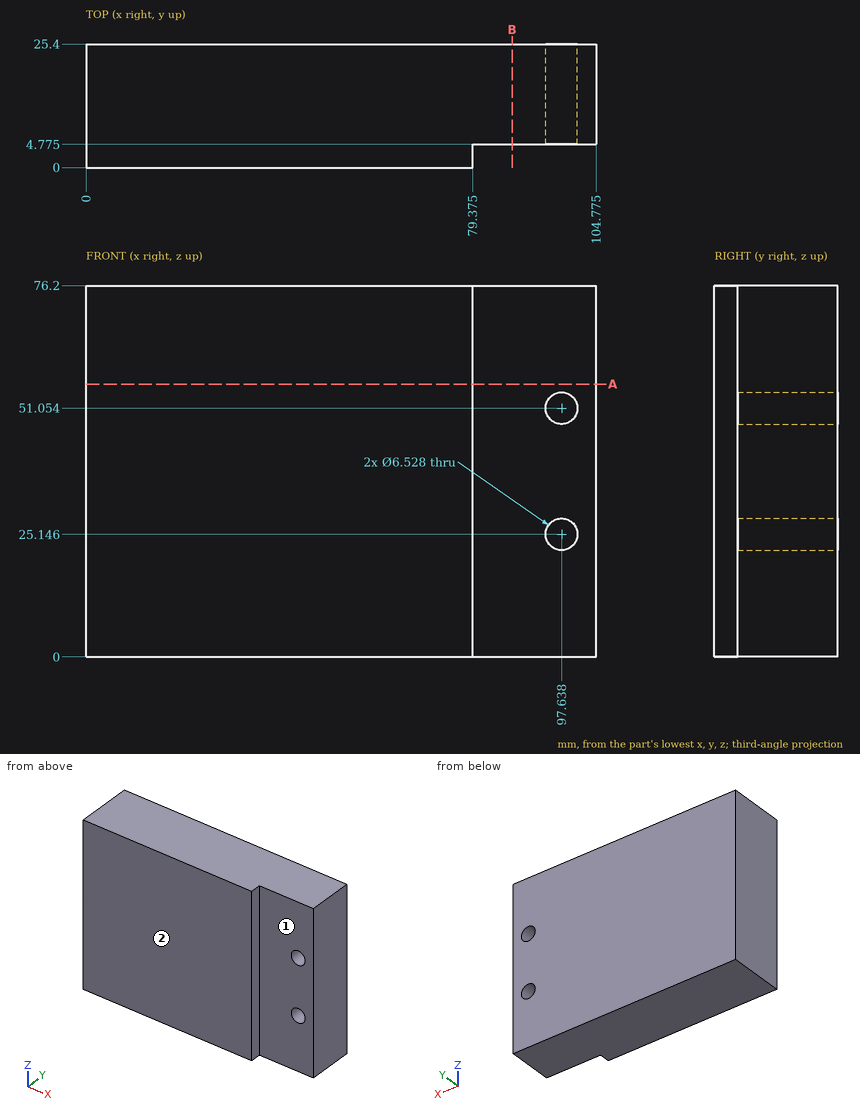
Job drawing, mm, ordinate dimensions from the low corner. One solid piece. A direction names the side the tool comes from. Give positions to 0.01 mm unless a question says otherwise; leave off trailing zeros. Loops run counter-clockwise (first coordinate to the right, second up) from the corner with the lowest first, then second, coordinate; pieces in that order, holes last. Notation, with made-up numbers: M -10.75,-21 L 0.25,-21 A19 cw 0.25,8 Z; hole C 9,-38.75 d7. An arc over 180 degrees is marked long. Return JSON: item names as keys, results as strings.
1) Flat gauge pins, fed straight in: pin 1 Ø8 at (x, y) = (74, 4.5) entering from -Z; pin 2 Ø7.5 at (x, z) = (96, 56) entering from -Y (1 decimal); pin 3 Ø2.5 at (y, z) = (3, 42) entering from +X (3 decimals). Where does each tip first touch, or does it go through?
Calculated:
{"pin 1": "stops at z = 0", "pin 2": "stops at y = 4.8", "pin 3": "stops at x = 79.375"}
2) Saw through at A-A, the plane z = 56. List the corners of the cut face in (x, y) (1 decimal), then the cut area to 3 significant figures.
Calculated:
{"outline": "M 0,0 L 79.4,0 L 79.4,4.8 L 104.8,4.8 L 104.8,25.4 L 0,25.4 Z", "area": "2,540 mm2"}
3) Saw through at B-B, the plane x = 87.5. List the corners of the cut face in (y, z) (1 decimal).
Calculated:
{"outline": "M 4.8,0 L 25.4,0 L 25.4,76.2 L 4.8,76.2 Z"}
4) Drill centre lines: line 1 (X direction, y = 24, z = 51) (1 decimal); line 2 (X direction, y = 4, z = 45) (1 decimal); line 3 (Y direction, x = 87.5, z = 30) (1 decimal). Where is each one in solid material? Low to high.
Calculated:
{"line 1": "x = 0 to 94.4, 100.9 to 104.8", "line 2": "x = 0 to 79.4", "line 3": "y = 4.8 to 25.4"}
5) 3-axis set-ups, long thin cutter, end or side, ignore diameter. For the marked faces 1 and 2: which of +Z, -Z, +X, -X, +Y, -Y reach the whole face in a straight line?
Calculated:
{"face 1": "+Z, -Z, +X, -Y", "face 2": "+Z, -Z, +X, -X, -Y"}
